Check sheet for the modelled part. Datum: model origin and axes. Units: mm. Round coordinates to 2 decimals unless told otherwise and drop trailing zeros. Write each loop counter-clockwise with the first axis right and the second up, starting at its lowest first coordinate (ties: lowest second). Pieces come first, ordered by that corner, then holes.
Item 1: Depth check by flat-ended pin: pin 1 (7 mm diameter, centred on x = 0, z = 37.5, fed in from -Y); pin 2 (2 mm diameter, centred on x = 0, z = 87.5, fed in from -Y); pin 3 (3 mm diameter, centred on x = -0.5, z = 311, fed in from +Y); pin 4 (1.8 mm diameter, centred on x = -1.5, z = 11.5, fed in from +Y). Enter the tip coordinate at first touch or a pass-through.
Item 2: Section check B-B, the plane z = 24. Record the cut outline in (x, y).
Item 3: Section check A-A, the plane y = -2. State how many separate pieces and enclosed holes the cut face has, plus the area to 3 significant figures.
Item 4: Material ranges on line 1 along X through (y, z) = (1.25, 87.5); line 2 along X through (y, z) = (2, 312.5); line 3 along Y through (x, z) = (-5.5, 279.5), recorded low to high.
from build123d import *

# Parameters (mm, degrees)
BOSS_EXTRUDE1_DEPTH = 350
CHAMFER1_SIZE       = 0.3
LPATTERN1_COUNT     = 14
LPATTERN1_PITCH     = 25


with BuildPart() as part:
    # Sketch1 → Boss-Extrude1 (new body)
    with BuildSketch(Plane.XY):
        with BuildLine():
            Line((-6, 4), (6, 4))
            Line((6, 4), (6, 2.75))
            Line((6, 2.75), (6, 2.559016994))
            ThreePointArc((6, 2.559016994), (5.706107374, 2.475528258), (5.5, 2.25))
            Line((5.5, 2.25), (5, 2.25))
            Line((5, 2.25), (5, 1.75))
            Line((5, 1.75), (5.5, 1.75))
            ThreePointArc((5.5, 1.75), (5.706107374, 1.524471742), (6, 1.440983006))
            Line((6, 1.440983006), (6, 1.25))
            Line((6, 1.25), (6, -4))
            Line((6, -4), (-6, -4))
            Line((-6, -4), (-6, 1.25))
            Line((-6, 1.25), (-6, 1.440983006))
            ThreePointArc((-6, 1.440983006), (-5.706107374, 1.524471742), (-5.5, 1.75))
            Line((-5.5, 1.75), (-5, 1.75))
            Line((-5, 1.75), (-5, 2.25))
            Line((-5, 2.25), (-5.5, 2.25))
            ThreePointArc((-5.5, 2.25), (-5.706107374, 2.475528258), (-6, 2.559016994))
            Line((-6, 2.559016994), (-6, 2.75))
            Line((-6, 2.75), (-6, 4))
        make_face()
    extrude(amount=BOSS_EXTRUDE1_DEPTH)

    # Chamfer1
    chamfer1_edges = [part.edges().sort_by_distance(p)[0] for p in [
        (-6, 4, 175),
        (6, 4, 175),
        (6, -4, 175),
        (-6, -4, 175),
    ]]
    chamfer(chamfer1_edges, length=CHAMFER1_SIZE)

    # Sketch3 → M3 六角承窩頭蓋螺釘的柱孔1 (revolve, cut)
    with BuildSketch(Plane(origin=(0, 4, 12.5), x_dir=(0, 0, 1), z_dir=(1, 0, 0))):
        Polygon((0, 0), (0, 8), (2, 8), (1.75, 7.75), (1.75, 4.5), (3, 4.5), (3, 0.5), (3.5, 0), align=None)
    hole_wizard_m3_1 = revolve(axis=Axis((0, 10.35, 12.5), (0, -1, 0)), mode=Mode.SUBTRACT)

    # LPattern1: M3 六角承窩頭蓋螺釘的柱孔1 ×14
    with Locations(*[(0, 0, i * LPATTERN1_PITCH) for i in range(1, LPATTERN1_COUNT)]):
        add(hole_wizard_m3_1, mode=Mode.SUBTRACT)


solid = part.part
Values found:
1. pin 1: stops at y = -4
1. pin 2: passes through
1. pin 3: stops at y = 3.58
1. pin 4: stops at y = -0.5
2. outline: (-6, -3.7) - (-5.7, -4) - (5.7, -4) - (6, -3.7) - (6, 1.44) arc R0.56 cw to (5.5, 1.75) - (5, 1.75) - (5, 2.25) - (5.5, 2.25) arc R0.56 cw to (6, 2.56) - (6, 3.7) - (5.7, 4) - (-5.7, 4) - (-6, 3.7) - (-6, 2.56) arc R0.56 cw to (-5.5, 2.25) - (-5, 2.25) - (-5, 1.75) - (-5.5, 1.75) arc R0.56 cw to (-6, 1.44) - close
3. separate pieces: 1
3. enclosed holes: 14
3. area: 4,070 mm2
4. line 1: x = -6 to -3, 3 to 6
4. line 2: x = -5 to -3, 3 to 5
4. line 3: y = -4 to 1.75, 2.25 to 4
